from build123d import *

# Parameters (mm, degrees)
F0_W     = 50.8
F0_H     = 101.6
F0_R     = 7.62
F1_DEPTH = 12.7
F2_R     = 5.08
F3_R     = 3.844677
F4_DEPTH = 25.4


with BuildPart() as f1:
    # F0 (on Front) → F1 (new body, symmetric)
    with BuildSketch(Plane.XZ):
        Rectangle(F0_W, F0_H)
        with Locations((0, -27.914425)):
            Circle(F0_R, mode=Mode.SUBTRACT)
        with Locations((0, 27.914425)):
            Circle(F0_R, mode=Mode.SUBTRACT)
    extrude(amount=F1_DEPTH, both=True)

    # F2
    f2_edges = [f1.edges().sort_by_distance(p)[0] for p in [
        (25.4, 0, 50.8),
        (25.4, 0, -50.8),
        (-25.4, 0, -50.8),
        (-25.4, 0, 50.8),
    ]]
    fillet(f2_edges, radius=F2_R)

    # F3 (on face) → F4 (cut)
    with BuildSketch(Plane.XZ.offset(12.7)):
        with Locations((-16.676344, 41.827552)):
            Circle(F3_R)
        with Locations((16.676344, 41.827552)):
            Circle(F3_R)
        with Locations((-16.676344, -41.827552)):
            Circle(F3_R)
        with Locations((16.676344, -41.827552)):
            Circle(F3_R)
    extrude(amount=-F4_DEPTH, mode=Mode.SUBTRACT)


solid = f1.part
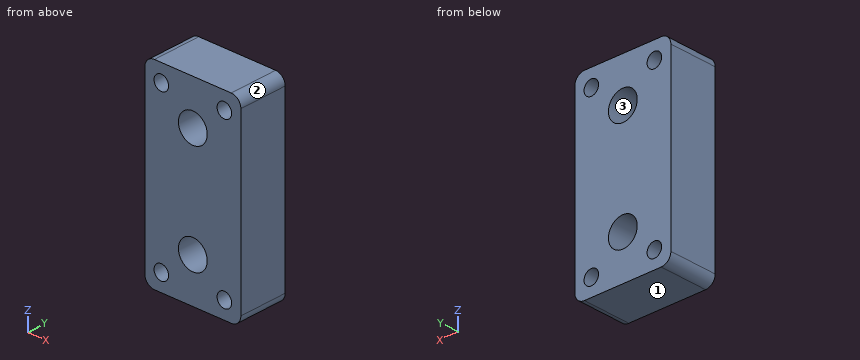
Design review of the part built by this model. Coordinates are the model's own, in mm. Face numbers are marked on the shaded views. Coordinates: 2 decimals unless noted, no trailing zeros. Loops run counter-clockwise (first coordinate to the right, second up) from the corner with the lowest first, then second, coordinate; pieces in that order, holes last. Notation, with made-up numbers: M 47.5,73 L 69.5,73 A9 ccw 69.5,82 Z; hole C 35,28 d3. An arc over 180 degrees is marked long. Use one line per item in the form item = value.
(1) For line 1 along Z through (x, y) = (16.5, -6.25); line 2 along Z through (x, y) = (15.5, -3.75); line 3 along X through (y, z) = (-5, -42.5), list the stretches that pass through material, from the lowest coordinate up. Write a range as from..to.
Return value:
line_1 = -50.8..-45.67, -37.99..37.99, 45.67..50.8
line_2 = -50.8..-45.49, -38.17..38.17, 45.49..50.8
line_3 = -25.4..-20.46, -12.89..12.89, 20.46..25.4
(2) Consider section A-A (x = 0). Write out the cut boundary in (y, z).
Return value:
outline = M -12.7,-50.8 L 12.7,-50.8 L 12.7,-35.53 L -12.7,-35.53 Z; M -12.7,-20.29 L 12.7,-20.29 L 12.7,20.29 L -12.7,20.29 Z; M -12.7,35.53 L 12.7,35.53 L 12.7,50.8 L -12.7,50.8 Z
(3) Consider section B-B (z = -23). Write out the cut boundary in (x, y), and give its area (3 significant figures).
Return value:
outline = M -25.4,-12.7 L -5.82,-12.7 L -5.82,12.7 L -25.4,12.7 Z; M 5.82,-12.7 L 25.4,-12.7 L 25.4,12.7 L 5.82,12.7 Z
area = 994 mm2
(4) Draft analysis for pull direction X (two halves, no side actions). For the marked faces 1, 2 and 3, state which applies: pulls with the +X half, pulls with the -X half, needs draft (parallel to the pull), parting line crosses it, or undercut.
Return value:
face_1 = needs draft
face_2 = pulls with the +X half
face_3 = undercut
(5) Clearance check with a flat-ended pin moving along its axis: P1, Ø20, axis at x = 0, z = 27.91, coming from the -Y side. State where the tip first meets the part, or that it passes through.
Return value:
P1 = -12.7
(6) Consider section D-D (y = 1.25). Write out the cut boundary in (x, z), and give its area (3 significant figures).
Return value:
outline = M -25.4,-45.72 A5.08 ccw -20.32,-50.8 L 20.32,-50.8 A5.08 ccw 25.4,-45.72 L 25.4,45.72 A5.08 ccw 20.32,50.8 L -20.32,50.8 A5.08 ccw -25.4,45.72 Z; hole C -16.68,-41.83 d7.69; hole C -16.68,41.83 d7.69; hole C 0,-27.91 d15.24; hole C 0,27.91 d15.24; hole C 16.68,-41.83 d7.69; hole C 16.68,41.83 d7.69
area = 4,590 mm2
(7) Consider section C-C (z = 43). Write out the cut boundary in (x, y).
Return value:
outline = M -25.4,-12.7 L -20.34,-12.7 L -20.34,12.7 L -25.4,12.7 Z; M -13.01,-12.7 L 13.01,-12.7 L 13.01,12.7 L -13.01,12.7 Z; M 20.34,-12.7 L 25.4,-12.7 L 25.4,12.7 L 20.34,12.7 Z
